Check sheet for the drawn part. Datum: minimum x, y, z corner. Units: mm. A direction names the side the tool comes from. Coordinates: 2 decimals unless noted, no trailing zeros. Loops run counter-clockwise (first coordinate to the right, second up) from the corner with the lowest first, then second, coordinate; pieces in that order, holes last.
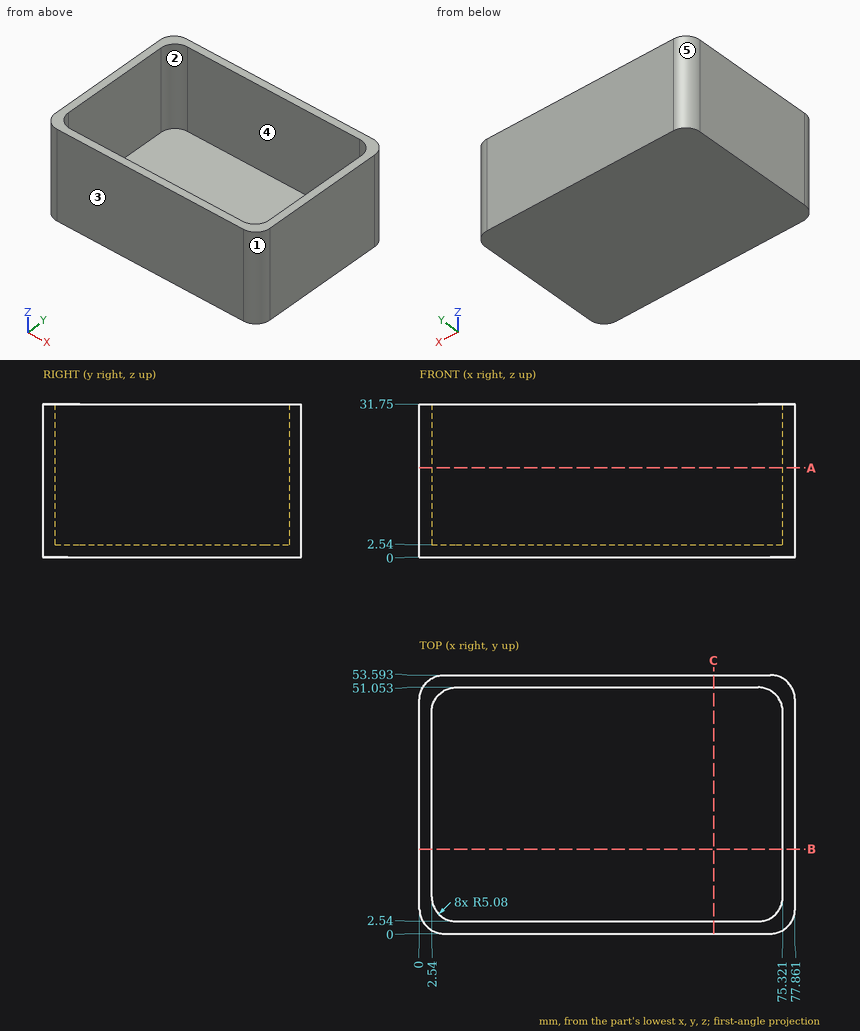
1) Section check B-B on y = 17.5. Enter the section's corners in (x, z).
Answer sheet:
outline: (0, 0) - (77.86, 0) - (77.86, 31.75) - (75.32, 31.75) - (75.32, 2.54) - (2.54, 2.54) - (2.54, 31.75) - (0, 31.75) - close
2) Depth check by flat-ended pin: pin 1 (10 mm diameter, centred on x = 42.5, z = 12, fed in from -Y); pin 2 (2 mm diameter, centred on x = 36, y = 19.5, fed in from +Z). Enter the tip coordinate at first touch or a pass-through.
Answer sheet:
pin 1: stops at y = 0
pin 2: stops at z = 2.54
3) Mould release check, pull along X, two halves, no side actions. Record for the marked faces 1, 2 and 3: +X half, -X half, draft (parallel to the pull), parting line (faces both ways), or undercut.
Answer sheet:
face 1: +X half
face 2: undercut
face 3: draft
4) Section check A-A on z = 18.5. Enter the section's corners in (x, y), plus the area to 3 significant figures.
Answer sheet:
outline: (0, 5.08) arc R5.08 ccw to (5.08, 0) - (72.78, 0) arc R5.08 ccw to (77.86, 5.08) - (77.86, 48.51) arc R5.08 ccw to (72.78, 53.59) - (5.08, 53.59) arc R5.08 ccw to (0, 48.51) - close; hole (2.54, 7.62) arc R5.08 ccw to (7.62, 2.54) - (70.24, 2.54) arc R5.08 ccw to (75.32, 7.62) - (75.32, 45.97) arc R5.08 ccw to (70.24, 51.05) - (7.62, 51.05) arc R5.08 ccw to (2.54, 45.97) - close
area: 642 mm2
5) Section check C-C on x = 61. Enter the section's corners in (y, z).
Answer sheet:
outline: (0, 0) - (53.59, 0) - (53.59, 31.75) - (51.05, 31.75) - (51.05, 2.54) - (2.54, 2.54) - (2.54, 31.75) - (0, 31.75) - close
6) Set-up check for the marked faces 4 and 5: record each of +Z, -Z, +X, -X, +Y, -Y from which the full face is reachable in a straight line by a thin tool's end or side.
Answer sheet:
face 4: +Z
face 5: +Z, -Z, -X, +Y
7) Scan lines: line 1 (Y direction, x = 56.5, z = 20); line 2 (X direction, y = 14.5, z = 6.5); line 3 (Z direction, x = 4, y = 25). Record each from-to range of solid material in increasing order.
Answer sheet:
line 1: y = 0 to 2.54, 51.05 to 53.59
line 2: x = 0 to 2.54, 75.32 to 77.86
line 3: z = 0 to 2.54
